The model under review builds one solid part; all positions refer to its coordinate system, in mm. A direction names the side the tool comes from. Coordinates: 2 decimals unless noted, no trailing zeros. Order: outer loops, then holes, each group sorted by start corner. A loop starts at its lowest first (then second) coordinate and runs counter-clockwise, first axis right, second up.
from build123d import *

# Parameters (mm, degrees)
F0_W     = 55.4
F0_H     = 41
F0_W_2   = 51.4
F0_H_2   = 37
F1_DEPTH = 15
F2_DEPTH = 2
F4_DEPTH = 41.001
F6_DEPTH = 55.401
F7_R     = 0.75


with BuildPart() as f1:
    # F0 (on Top) → F1 (new body)
    with BuildSketch(Plane.XY):
        Rectangle(F0_W, F0_H)
        Rectangle(F0_W_2, F0_H_2, mode=Mode.SUBTRACT)
    extrude(amount=F1_DEPTH)

    # F0 (on Top) → F2 (join)
    with BuildSketch(Plane.XY):
        Rectangle(F0_W, F0_H)
        Rectangle(F0_W_2, F0_H_2, mode=Mode.SUBTRACT)
        Rectangle(F0_W_2, F0_H_2)
    extrude(amount=-F2_DEPTH)

    # F3 (on face) → F4 (cut, through all)
    with BuildSketch(Plane.XZ.offset(20.5)):
        Polygon((19.7, 15), (-19.7, 15), (-14, 6), (14, 6), align=None)
    extrude(amount=-F4_DEPTH, mode=Mode.SUBTRACT)

    # F5 (on face) → F6 (cut, through all)
    with BuildSketch(Plane(origin=(-27.7, 0, 0), x_dir=(0, -1, 0), z_dir=(-1, 0, 0))):
        Polygon((12.5, 15), (-12.5, 15), (-8.0000100486, 6), (8.0000100486, 6), align=None)
    extrude(amount=-F6_DEPTH, mode=Mode.SUBTRACT)

    # F7
    f7_edges = [f1.edges().sort_by_distance(p)[0] for p in [
        (0, 20.5, 6),
        (16.85, 20.5, 10.5),
        (23.7, 20.5, 15),
        (27.7, 16.5, 15),
        (27.7, 20.5, 6.5),
        (-16.85, 20.5, 10.5),
        (-23.7, 20.5, 15),
        (-27.7, 20.5, 6.5),
        (-27.7, 16.5, 15),
        (-25.7, 15.5, 15),
        (-22.7, 18.5, 15),
        (-16.85, 18.5, 10.5),
        (0, 18.5, 6),
        (16.85, 18.5, 10.5),
        (22.7, 18.5, 15),
        (25.7, 15.5, 15),
        (26.7, 12.5, 15),
        (27.7, 10.250005, 10.5),
        (25.7, 10.250005, 10.5),
        (25.7, 0, 6),
        (27.7, 0, 6),
        (27.7, -10.250005, 10.5),
        (25.7, -10.250005, 10.5),
        (26.7, -12.5, 15),
        (27.7, -16.5, 15),
        (25.7, -15.5, 15),
        (22.7, -18.5, 15),
        (23.7, -20.5, 15),
        (27.7, -20.5, 6.5),
        (19.7, -19.5, 15),
        (16.85, -18.5, 10.5),
        (16.85, -20.5, 10.5),
        (0, -20.5, 6),
        (0, -18.5, 6),
        (-16.85, -18.5, 10.5),
        (-16.85, -20.5, 10.5),
        (-19.7, -19.5, 15),
        (-22.7, -18.5, 15),
        (-23.7, -20.5, 15),
        (-25.7, -15.5, 15),
        (-26.7, -12.5, 15),
        (-27.7, -16.5, 15),
        (-25.7, -10.250005, 10.5),
        (-27.7, -10.250005, 10.5),
        (-26.7, 12.5, 15),
        (-27.7, 0, 6),
        (-25.7, 0, 6),
        (-25.7, 10.250005, 10.5),
        (-27.7, 10.250005, 10.5),
        (-27.7, -20.5, 6.5),
        (-27.7, 0, -2),
        (0, 20.5, -2),
        (0, -20.5, -2),
        (27.7, 0, -2),
    ]]
    fillet(f7_edges, radius=F7_R)


solid = f1.part
(1) Consider section A-A (z = 2.5). Give the boundary of the cut face in (x, y), then the cut area to 3 significant figures.
(2) Consider section C-C (x = -6). Give the boundary of the cut face in (y, z), then the cut area to 3 significant figures.
(3) Tool access review of faces 1 (the face through (16.81, 19.5, 10.44)), 2 (the face through (16.972, 20.286, 10.27)), 3 (the face through (0, 0, 0)), 4 (the face through (26.7, -10.1, 10.2)): name each direction out of +Z, -Z, +X, -X, +Y, -Y from which nothing blocks a thin tool from reaching the whole face with its end or side.
(4) Consider section B-B (y = 15.5). Give the boundary of the cut face in (x, z), then the cut area to 3 significant figures.
(5) Consider section D-D (z = 9.25). Give the number of separate pieces and of enclosed holes in the cut face, then the cut area to 3 significant figures.
(6) Insertion check: pin 1 Ø0.6 at (x, y) = (0, -19.5) entering from +Z; pin 2 Ø8 at (x, y) = (-7, -2) entering from +Z. Each pin has a flat end and moves straight along its axis. Give the tip position at first contact, or say it passes through.
(7) The part is to be moulded in two halves that separate along X. For faces 5 (the face through (-27.486, 10.213, 9.922)), 6 (the face through (26.7, 10.2, 10.4)), 7 (the face through (0, -18.5, 4)), say which applies: +X half, -X half, draft (parallel to the pull), parting line (faces both ways), or undercut.
(8) Wall thickness on line 1 (Y direction, x = 20, z = 4); line 2 (X direction, y = -1, z = 4.5); line 3 (Z direction, x = -6, y = -16): over which ranges is each line inside the solid? List them lowest first.
Findings:
1. outline: (-27.7, -19.75) arc R0.75 ccw to (-26.95, -20.5) - (26.95, -20.5) arc R0.75 ccw to (27.7, -19.75) - (27.7, 19.75) arc R0.75 ccw to (26.95, 20.5) - (-26.95, 20.5) arc R0.75 ccw to (-27.7, 19.75) - close; hole (-25.7, -18.5) - (25.7, -18.5) - (25.7, 18.5) - (-25.7, 18.5) - close
1. area: 369 mm2
2. outline: (-20.5, -1.25) arc R0.75 ccw to (-19.75, -2) - (19.75, -2) arc R0.75 ccw to (20.5, -1.25) - (20.5, 5.25) arc R0.75 ccw to (19.75, 6) - (19.25, 6) arc R0.75 ccw to (18.5, 5.25) - (18.5, 0) - (-18.5, 0) - (-18.5, 5.25) arc R0.75 ccw to (-19.25, 6) - (-19.75, 6) arc R0.75 ccw to (-20.5, 5.25) - close
2. area: 105 mm2
3. face 1: +Z, +Y, -Y
3. face 2: +Z, +Y
3. face 3: +Z
3. face 4: +Z, +X, -X
4. outline: (-27.7, -1.25) arc R0.75 ccw to (-26.95, -2) - (26.95, -2) arc R0.75 ccw to (27.7, -1.25) - (27.7, 14.25) arc R0.75 ccw to (26.95, 15) - (26.45, 15) arc R0.75 ccw to (25.7, 14.25) - (25.7, 0) - (-25.7, 0) - (-25.7, 14.25) arc R0.75 ccw to (-26.45, 15) - (-26.95, 15) arc R0.75 ccw to (-27.7, 14.25) - close
4. area: 170 mm2
5. separate pieces: 4
5. enclosed holes: 0
5. area: 161 mm2
6. pin 1: stops at z = 6
6. pin 2: stops at z = 0
7. face 5: -X half
7. face 6: draft
7. face 7: undercut
8. line 1: y = -20.5 to -18.5, 18.5 to 20.5
8. line 2: x = -27.7 to -25.7, 25.7 to 27.7
8. line 3: z = -2 to 0
